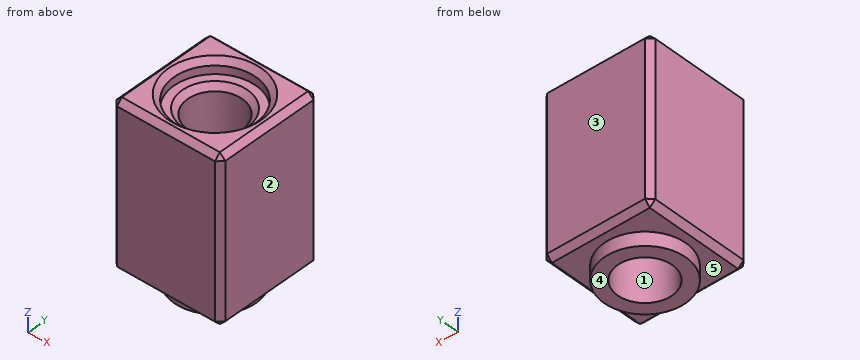
from build123d import *

# Parameters (mm, degrees)
F0_W     = 40
F0_H     = 40
F1_DEPTH = 60
F2_R     = 15
F3_DEPTH = 60
F5_START = -5
F4_R     = 15
F4_R_2   = 10
F5_DEPTH = 60
F6_SIZE  = 2


with BuildPart() as f1:
    # F0 (on Top) → F1 (new body)
    with BuildSketch(Plane.XY):
        Rectangle(F0_W, F0_H)
    extrude(amount=F1_DEPTH)

    # F2 (on face) → F3 (cut, through all)
    with BuildSketch(Plane.XY.offset(60)):
        Circle(F2_R)
    extrude(amount=-F3_DEPTH, mode=Mode.SUBTRACT)

    # F4 (on face) → F5 (join)
    with BuildSketch(Plane.XY.offset(60).offset(F5_START)):
        Circle(F4_R)
        Circle(F4_R_2, mode=Mode.SUBTRACT)
    extrude(amount=-F5_DEPTH)

    # F6
    f6_edges = [f1.edges().sort_by_distance(p)[0] for p in [
        (-20, -20, 30),
        (20, -20, 30),
        (0, -20, 60),
        (0, -20, 0),
        (20, 0, 0),
        (20, 20, 30),
        (20, 0, 60),
        (-20, 0, 60),
        (0, 20, 60),
        (-20, 20, 30),
        (-20, 0, 0),
        (0, 20, 0),
        (-15, 0, 60),
        (-10, 0, 55),
    ]]
    chamfer(f6_edges, length=F6_SIZE)


solid = f1.part
Design review of the part built by this model. Coordinates are the model's own, in mm. Face numbers are marked on the shaded views. A direction names the side the tool comes from. Round coordinates to 2 decimals unless told otherwise and drop trailing zeros. Write each loop counter-clockwise with the first axis right and the second up, starting at its lowest first coordinate (ties: lowest second). Pieces come first, ordered by that corner, then holes. Notation, with made-up numbers: (29, 76.25) -> (56, 76.25) arc R16 ccw to (56, 98.25) -> close; hole circle Ø11 at (78, -34.75). An arc over 180 degrees is marked (long way). One line per item, written item: value. Start each with the question number.
Q1. Add section B-B (z = 34). Give the boundary of the cut face in (x, y).
Q2. To check wall thickness, follow probe 1 along Y at (x, z) = (0, 56.2); probe 2 along Y at (x, z) = (0, 8); probe 3 along Z at (x, y) = (-17, 13). State the ranges of each line that lie inside material, in increasing order.
Q3. Add section A-A (x = 0). Give the boundary of the cut face in (y, z), then the cut area to 3 significant figures.
Q4. Tool access review of the marked faces 4 and 5: name each direction out of +Z, -Z, +X, -X, +Y, -Y from which nothing blocks a thin tool from reaching the whole face with its end or side.
Q5. Insertion check: P1, Ø24, axis at x = -5.5, y = 0.5, coming from the +Z side; P2, Ø6, axis at x = 7, y = -1, coming from the +Z side. Each pin has a flat end and moves straight along its axis. Give the tip position at first contact, or say it passes through.
Q6. The part is to be moulded in two halves that separate along Y. For the marked faces 1, 2 and 3, say which applies: pulls with the +Y half, pulls with the -Y half, needs draft (parallel to the pull), parting line crosses it, or undercut.
Response:
1. outline: (-20, -18) -> (-18, -20) -> (18, -20) -> (20, -18) -> (20, 18) -> (18, 20) -> (-18, 20) -> (-20, 18) -> close; hole circle Ø20 at (0, 0)
2. probe 1: y = -20 to -15, 15 to 20
2. probe 2: y = -20 to -10, 10 to 20
2. probe 3: z = 0 to 60
3. outline: (-20, 2) -> (-18, 0) -> (-15, 0) -> (-15, -5) -> (-10, -5) -> (-10, 53) -> (-12, 55) -> (-15, 55) -> (-15, 58) -> (-17, 60) -> (-18, 60) -> (-20, 58) -> close; (10, -5) -> (15, -5) -> (15, 0) -> (18, 0) -> (20, 2) -> (20, 58) -> (18, 60) -> (17, 60) -> (15, 58) -> (15, 55) -> (12, 55) -> (10, 53) -> close
3. area: 1,180 mm^2
4. face 4: -Z, +X, -X, +Y, -Y
4. face 5: -Z
5. P1: stops at z = 60
5. P2: stops at z = 53.07
6. face 1: undercut
6. face 2: needs draft
6. face 3: pulls with the +Y half
